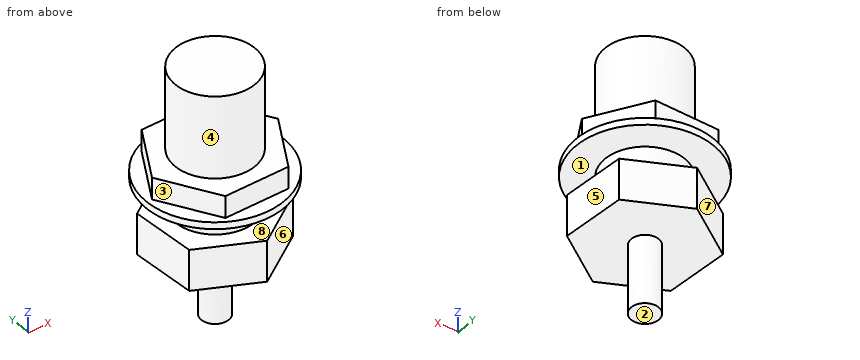
from build123d import *

# Parameters (mm, degrees)
SKETCH1_R           = 2.9
BOSS_EXTRUDE1_DEPTH = 3
BOSS_EXTRUDE2_DEPTH = 1.6
SKETCH3_R           = 5
BOSS_EXTRUDE3_DEPTH = 0.5
SKETCH4_R           = 2.9
BOSS_EXTRUDE4_DEPTH = 2
BOSS_EXTRUDE5_DEPTH = 3
SKETCH6_R           = 1
BOSS_EXTRUDE6_DEPTH = 5


with BuildPart() as part:
    # Sketch1 → Boss-Extrude1 (new, symmetric)
    with BuildSketch(Plane.XY):
        Circle(SKETCH1_R)
    extrude(amount=BOSS_EXTRUDE1_DEPTH, both=True)

    # Sketch2 → Boss-Extrude2 (add)
    with BuildSketch(Plane(origin=(0, 0, -3), x_dir=(-1, 0, 0), z_dir=(0, 0, -1))):
        Polygon((4.618802154, 0), (2.309401077, 4), (-2.309401077, 4), (-4.618802154, 0), (-2.309401077, -4), (2.309401077, -4), align=None)
    extrude(amount=BOSS_EXTRUDE2_DEPTH)

    # Sketch3 → Boss-Extrude3 (add)
    with BuildSketch(Plane(origin=(0, 0, -4.6), x_dir=(-1, 0, 0), z_dir=(0, 0, -1))):
        Circle(SKETCH3_R)
    extrude(amount=BOSS_EXTRUDE3_DEPTH)

    # Sketch4 → Boss-Extrude4 (add)
    with BuildSketch(Plane(origin=(0, 0, -5.1), x_dir=(-1, 0, 0), z_dir=(0, 0, -1))):
        with Locations(Location((0, 0, 0), (0, 0, 180))):
            Circle(SKETCH4_R)
    extrude(amount=BOSS_EXTRUDE4_DEPTH)

    # Sketch5 → Boss-Extrude5 (add)
    with BuildSketch(Plane(origin=(0, 0, -7.1), x_dir=(-1, 0, 0), z_dir=(0, 0, -1))):
        Polygon((4.134382211, 2.059178737), (0.283890008, 4.610069392), (-3.850492202, 2.550890655), (-4.134382211, -2.059178737), (-0.283890008, -4.610069392), (3.850492202, -2.550890655), align=None)
    extrude(amount=BOSS_EXTRUDE5_DEPTH)

    # Sketch6 → Boss-Extrude6 (add)
    with BuildSketch(Plane(origin=(0, 0, -10.1), x_dir=(-1, 0, 0), z_dir=(0, 0, -1))):
        Circle(SKETCH6_R)
    extrude(amount=BOSS_EXTRUDE6_DEPTH)


solid = part.part
Work out the finished part from the listing and answer in its coordinate system (mm). Face numbers are marked on the shaded views. A direction names the side the tool comes from. Coordinates: 2 decimals unless noted, no trailing zeros. Write each loop counter-clockwise with the first axis right and the second up, starting at its lowest first coordinate (ties: lowest second). Pieces come first, ordered by that corner, then holes. Notation, with made-up numbers: M -24.5,38.25 L 10.5,38.25 A21 ccw 10.5,68.25 Z; hole C 36.25,18 d11. An arc over 180 degrees is marked long. Use one line per item in the form item = value. Start each with the question number.
1. A tool of negligible diameter and unlimited length cuts with its end or side. For the marked faces 4, 5, 6, 7 and 8, from which of +Z, -Z, +X, -X, +Y, -Y can it reach the whole face along a straight path? Write none if from no direction.
2. Straight lines are drawn through the part: probe 1 along Z at (x, y) = (-3, -2); probe 2 along Z at (x, y) = (-3.5, -2.5); probe 3 along Z at (x, y) = (1.75, 0.25). For each, find the intervals that lie inside material, in ascending order. Write a range as from..to.
3. The part is cut by section A-A (y = -3.25). Give the vertices of the cut face in (x, z), plus the area to 3 significant figures.
4. Each of these flat-tipped pins is pushed along its axis until it touches: P1, Ø5, axis at x = 4, z = -8.5, coming from the -Y side; P2, Ø2.5, axis at x = 2, y = -1.5, coming from the -Z side; P3, Ø6, axis at x = 2.5, z = -1, coming from the +Y side. Where does it stop, or does it pass through?
5. The mould has two halves that part along Z. Classify the marked faces 1, 2 and 3: released by +Z, released by -Z, zero draft, split by the parting line, or undercut.
6. The part is cut by section D-D (z = -12.75). Give the vertices of the cut face in (x, y).
7. The part is cut by section B-B (x = 3.5). Give the vertices of the cut face in (y, z), plus the area to 3 significant figures.
8. The part is cut by section C-C (x = 2.5). Give the vertices of the cut face in (y, z), plus the area to 3 significant figures.
Evaluation:
q1.face_4 = +Z
q1.face_5 = -Z, +X, +Y
q1.face_6 = -Z, +X, -Y
q1.face_7 = -Z, -X, +Y
q1.face_8 = none
q2.probe_1 = -10.1..-7.1, -5.1..-3
q2.probe_2 = -10.1..-7.1, -5.1..-4.6
q2.probe_3 = -10.1..3
q3.outline = M -3.8,-5.1 L 3.8,-5.1 L 3.8,-4.6 L 2.74,-4.6 L 2.74,-3 L -2.74,-3 L -2.74,-4.6 L -3.8,-4.6 Z; M -2.45,-10.1 L 2.34,-10.1 L 2.34,-7.1 L -2.45,-7.1 Z
q3.area = 26.9 mm^2
q4.P1 = -3.8
q4.P2 = -10.1
q4.P3 = 4
q5.face_1 = undercut
q5.face_2 = released by -Z
q5.face_3 = zero draft
q6.outline = C 0,0 d2
q7.outline = M -3.57,-5.1 L 3.57,-5.1 L 3.57,-4.6 L 1.94,-4.6 L 1.94,-3 L -1.94,-3 L -1.94,-4.6 L -3.57,-4.6 Z; M -2.48,-10.1 L 2.73,-10.1 L 2.73,-7.1 L -2.48,-7.1 Z
q7.area = 25.4 mm^2
q8.outline = M -4.33,-5.1 L -1.47,-5.1 L -1.47,-7.1 L -3.14,-7.1 L -3.14,-10.1 L 3.22,-10.1 L 3.22,-7.1 L 1.47,-7.1 L 1.47,-5.1 L 4.33,-5.1 L 4.33,-4.6 L 3.67,-4.6 L 3.67,-3 L 1.47,-3 L 1.47,3 L -1.47,3 L -1.47,-3 L -3.67,-3 L -3.67,-4.6 L -4.33,-4.6 Z
q8.area = 58.7 mm^2
